```python
from build123d import *

# Parameters (mm, degrees)
F1_DEPTH = 12


with BuildPart() as f1:
    # F0 (on Top) → F1 (new body)
    with BuildSketch(Plane.XY):
        with BuildLine():
            ThreePointArc((-2.542081, 3.088337), (3.617204, -1.707582), (-4, 0))
            Line((-4, 0), (-4, 2.288375))
            Line((-4, 2.288375), (-6.763066, 2.288375))
            Line((-6.763066, 2.288375), (-7.895562, -1.667487))
            Line((-7.895562, -1.667487), (-5.755623, -1.667487))
            Line((-5.755623, -1.667487), (-5.755623, -6))
            Line((-5.755623, -6), (6.164354, -6))
            Line((6.164354, -6), (5.840028, 6))
            Line((5.840028, 6), (-8.637475, 6))
            Line((-8.637475, 6), (-8.637475, 0.512484))
            ThreePointArc((-8.637475, 0.512484), (-12.637475, -3.487516), (-16.637475, 0.512484))
            Line((-16.637475, 0.512484), (-17.216573, 0.512484))
            Line((-17.216573, 0.512484), (-17.216573, -4.205178))
            Line((-17.216573, -4.205178), (-8.637475, -4.205178))
            Line((-8.637475, -4.205178), (-6.16524, -4.227431))
            Line((-6.16524, -4.227431), (-6.16524, -2.048139))
            Line((-6.16524, -2.048139), (-8.411505, -2.048139))
            Line((-8.411505, -2.048139), (-7.701935, 0.512484))
            Line((-7.701935, 0.512484), (-6.964513, 3.088337))
            Line((-6.964513, 3.088337), (-2.542081, 3.088337))
        make_face()
    extrude(amount=F1_DEPTH)


solid = f1.part
```
Part model, mm, in its own coordinate system. A direction names the side the tool comes from. Round coordinates to 2 decimals unless told otherwise and drop trailing zeros. Order: outer loops, then holes, each group sorted by start corner. A loop starts at its lowest first (then second) coordinate and runs counter-clockwise, first axis right, second up. Notation, with made-up numbers: M -17,45 L 38,45 A25 ccw 38,61 Z; hole C 51,65 d9. An arc over 180 degrees is marked long. Put each result on its own line as item: value. Start each with the question number.
1. Slice it at B-B on y = -3.75. List the corners of the cut face in (x, z), then the cut area to 3 significant figures.
2. Drill centre lines: probe 1 along Y at (x, z) = (0, 9.25); probe 2 along X at (y, z) = (-1.75, 3.5); probe 3 along Y at (x, z) = (-4.5, 2.5). Where is each one in solid material? Low to high. Write a range as [from, to].
3. Slice it at C-C on z = 10. List the corners of the cut face in (x, y).
4. Slice it at D-D on x = -5.5. List the corners of the cut face in (y, z), then the cut area to 3 significant figures.
5. Slice it at A-A on x = 0. List the corners of the cut face in (y, z).
6. Two-plate mould, pull along X, no slides. Class faces 6 (the face through (-8.637, 3, 6)), 7 (the face through (-1, 6, 6)), 8 (the face through (-12.55, -3.487, 5.916)): +X half, -X half, draft (parallel to the pull), parting line (faces both ways), or undercut.
7. Tool access for faces 1 (the face through (-6.165, -3, 6)), 2 (the face through (-7.34, 1.78, 5.92)), 3 (the face through (-13, -4.205, 6)), 4 (the face through (-3, -3, 0)), 5 (the face through (0, -6, 6)): list every direction of +Z, -Z, +X, -X, +Y, -Y with a clear straight run to the whole face (end or side of a thin tool).
8. Drop flat-ended pins along their axis: pin 1 (1.8 mm diameter, centred on y = 1, z = 3.5, fed in from +X); pin 2 (4.5 mm diameter, centred on y = 2, z = 3, fed in from -X); pin 3 (1.1 mm diameter, centred on y = -3, z = 6, fed in from +X); pin 4 (3 mm diameter, centred on x = -14, z = 1.5, fed in from +Y). Give the stop position or say it passes through.
Findings:
1. outline: M -17.22,0 L -6.17,0 L -6.17,12 L -17.22,12 Z; M -5.76,0 L -1.39,0 L -1.39,12 L -5.76,12 Z; M 1.39,0 L 6.1,0 L 6.1,12 L 1.39,12 Z
1. area: 242 mm2
2. probe 1: [-6, -4], [4, 6]
2. probe 2: [-17.22, -15.94], [-9.34, -8.33], [-5.76, -3.6], [3.6, 6.05]
2. probe 3: [-6, 2.29], [3.09, 6]
3. outline: M -17.22,-4.21 L -8.64,-4.21 L -6.17,-4.23 L -6.17,-2.05 L -8.41,-2.05 L -7.7,0.51 L -6.96,3.09 L -2.54,3.09 A4 cw long -4,0 L -4,2.29 L -6.76,2.29 L -7.9,-1.67 L -5.76,-1.67 L -5.76,-6 L 6.16,-6 L 5.84,6 L -8.64,6 L -8.64,0.51 A4 cw -16.64,0.51 L -17.22,0.51 Z
4. outline: M -6,0 L 2.29,0 L 2.29,12 L -6,12 Z; M 3.09,0 L 6,0 L 6,12 L 3.09,12 Z
4. area: 134 mm2
5. outline: M -6,0 L -4,0 L -4,12 L -6,12 Z; M 4,0 L 6,0 L 6,12 L 4,12 Z
6. face 6: -X half
6. face 7: draft
6. face 8: undercut
7. face 1: +Z, -Z, -Y
7. face 2: +Z, -Z
7. face 3: +Z, -Z, -X, -Y
7. face 4: -Z, +X, -X, +Y, -Y
7. face 5: +Z, -Z, +X, -X, -Y
8. pin 1: x = 6
8. pin 2: x = -17.22
8. pin 3: x = 6.1
8. pin 4: y = -2.28
